Read the model definition and answer for the solid it produces. Units are mm, in the model's axes. Give positions to 0.01 mm unless a question says otherwise; leave off trailing zeros. Order: outer loops, then holes, each group sorted by start corner. A loop starts at its lowest first (then second) coordinate and runs counter-clockwise, first axis right, second up.
Item 1: A cutting plane is placed at C-C (z = 4.4). State how many separate pieces and enclosed holes the cut face has, plus the area to 3 significant figures.
Item 2: A cutting plane is placed at B-B (x = -38.5). Write down the section's boundary in (y, z).
Item 3: A cutting plane is placed at A-A (y = -11). Write down the section's boundary in (x, z).
Item 4: Find the intervals of material crossed by line 1 along X through (y, z) = (11, 2.85); line 2 along Y through (x, z) = (-18, 2); line 3 along Y through (x, z) = (-27.5, 0.9), in increasing order.
from build123d import *

# Parameters (mm, degrees)
SKETCH1_W           = 57.15
SKETCH1_H           = 64.060512242
SKETCH1_R           = 3.175
SKETCH1_W_2         = 5.9944
SKETCH1_H_2         = 6.35
BOSS_EXTRUDE1_DEPTH = 5.9944


with BuildPart() as part:
    # Sketch1 → Boss-Extrude1 (new body)
    with BuildSketch(Plane(origin=(0, 0, 0), x_dir=(-1, 0, 0), z_dir=(0, 0, 1))):
        with Locations((33.534836058, -1.33105998)):
            Rectangle(SKETCH1_W, SKETCH1_H)
        with Locations((53.129579937, -24.38105998)):
            Circle(SKETCH1_R, mode=Mode.SUBTRACT)
        with Locations((53.129579937, 21.71894002)):
            Circle(SKETCH1_R, mode=Mode.SUBTRACT)
        with Locations((27.729579937, -24.38105998)):
            Circle(SKETCH1_R, mode=Mode.SUBTRACT)
        with Locations((27.729579937, 21.71894002)):
            Circle(SKETCH1_R, mode=Mode.SUBTRACT)
        with Locations((37.076779937, -8.707018437)):
            Rectangle(SKETCH1_W_2, SKETCH1_H_2, mode=Mode.SUBTRACT)
        Polygon((15.029579937, 13.517981563), (21.023979937, 13.517981563), (21.023979937, 7.36894002), (21.023979937, 7.167981563), (15.029579937, 7.167981563), (15.029579937, 7.36894002), align=None, mode=Mode.SUBTRACT)
        with Locations((18.026779937, -8.707018437)):
            Rectangle(SKETCH1_W_2, SKETCH1_H_2, mode=Mode.SUBTRACT)
        Polygon((40.073979937, 7.36894002), (40.073979937, 7.167981563), (34.079579937, 7.167981563), (34.079579937, 7.36894002), (34.079579937, 13.517981563), (40.073979937, 13.517981563), align=None, mode=Mode.SUBTRACT)
    extrude(amount=BOSS_EXTRUDE1_DEPTH)


solid = part.part
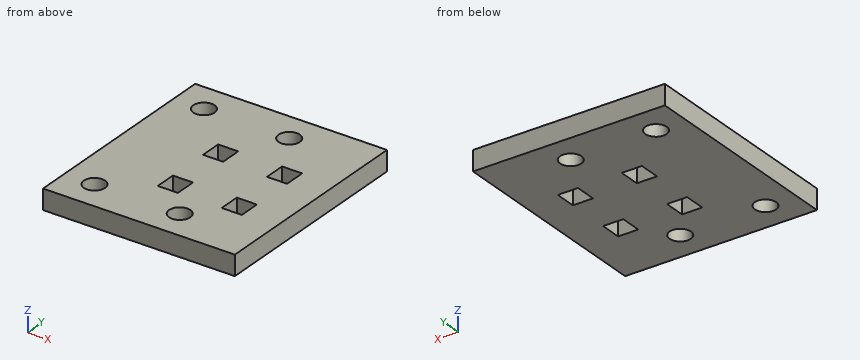
Response values:
1. separate pieces: 1
1. enclosed holes: 8
1. area: 3,380 mm2
2. outline: (-30.7, 0) - (-13.52, 0) - (-13.52, 5.99) - (-30.7, 5.99) - close; (-7.17, 0) - (5.53, 0) - (5.53, 5.99) - (-7.17, 5.99) - close; (11.88, 0) - (33.36, 0) - (33.36, 5.99) - (11.88, 5.99) - close
3. outline: (-62.11, 0) - (-40.07, 0) - (-40.07, 5.99) - (-62.11, 5.99) - close; (-34.08, 0) - (-21.02, 0) - (-21.02, 5.99) - (-34.08, 5.99) - close; (-15.03, 0) - (-4.96, 0) - (-4.96, 5.99) - (-15.03, 5.99) - close
4. line 1: x = -62.11 to -40.07, -34.08 to -21.02, -15.03 to -4.96
4. line 2: y = -30.7 to -13.52, -7.17 to 5.53, 11.88 to 33.36
4. line 3: y = -30.7 to -24.89, -18.55 to 21.21, 27.55 to 33.36
